```python
from build123d import *

# Parameters (mm, degrees)
SALIENTE_EXTRUIR1_DEPTH = 20
CORTAR_EXTRUIR1_DEPTH   = 20
CROQUIS3_W              = 4
CROQUIS3_H              = 20
SALIENTE_EXTRUIR2_DEPTH = 5


with BuildPart() as part:
    # Croquis1 → Saliente-Extruir1 (new body)
    with BuildSketch(Plane(origin=(0, 0, 0), x_dir=(1, 0, 0), z_dir=(0, 1, 0))):
        Polygon((-5, 19), (-2, 19), (-2, 3), (2, 3), (2, 19), (26, 19), (26, 16), (5, 16), (5, 0), (-5, 0), align=None)
    extrude(amount=SALIENTE_EXTRUIR1_DEPTH)

    # Croquis2 → Cortar-Extruir1 (cut)
    with BuildSketch(Plane.XY.offset(-16)):
        with BuildLine():
            Line((21.5, 16.5), (9.5, 16.5))
            ThreePointArc((9.5, 16.5), (8, 15), (9.5, 13.5))
            Line((9.5, 13.5), (21.5, 13.5))
            ThreePointArc((21.5, 13.5), (23, 15), (21.5, 16.5))
        make_face()
        with BuildLine():
            Line((21.5, 3.5), (9.5, 3.5))
            ThreePointArc((9.5, 3.5), (8, 5), (9.5, 6.5))
            Line((9.5, 6.5), (21.5, 6.5))
            ThreePointArc((21.5, 6.5), (23, 5), (21.5, 3.5))
        make_face()
    extrude(amount=-CORTAR_EXTRUIR1_DEPTH, mode=Mode.SUBTRACT)

    # Croquis3 → Saliente-Extruir2 (add)
    with BuildSketch(Plane(origin=(-2, 0, 0), x_dir=(0, 0, -1), z_dir=(1, 0, 0))):
        with Locations((17, 10)):
            Rectangle(CROQUIS3_W, CROQUIS3_H)
    extrude(amount=SALIENTE_EXTRUIR2_DEPTH)


solid = part.part
```
CAD build for the part. Positions are in the model's coordinates, mm. A direction names the side the tool comes from. Coordinates: 2 decimals unless noted, no trailing zeros. Order: outer loops, then holes, each group sorted by start corner. A loop starts at its lowest first (then second) coordinate and runs counter-clockwise, first axis right, second up. Notation, with made-up numbers: (32, 19) -> (51, 19) arc R24 ccw to (51, 58) -> close; hole circle Ø8 at (-39.75, -16). An arc over 180 degrees is marked (long way). Use one line per item in the form item = value. Start each with the question number.
1) Drop flat-ended pins along their axis: pin 1 (10 mm diameter, centred on x = 14.5, y = 8, fed in from +Z); pin 2 (5 mm diameter, centred on y = 7, z = -11.5, fed in from +X). Give the stop position or say it passes through.
2) Tool access for faces 1 (the flat face through (0, 10, -15)), 2 (the flat face through (16, 10, -16)), 3 (the flat face through (15, 6.5, -17)): list every direction of +Z, -Z, +X, -X, +Y, -Y with a clear straight run to the whole face (end or side of a thin tool).
3) Pull direction X, two halves, no side cores. Call faces 4 (the flat face through (-5, 10, -9)), 5 (the flat face through (15, 13.5, -17)), 6 (the flat face through (26, 10, -18)): +X half, -X half, draft (parallel to the pull), parting line (faces both ways), or undercut.
4) Drill centre lines: L1, parallel to X at y = 5, z = -8.5; L2, parallel to Z at x = -0.5, y = 1; L3, parallel to X at y = 13.5, z = -2. Where is each one in solid material? Low to high. Write a range as [from, to].
5) Band-saw the part on C-C on x = 15. Give the cut face in (y, z).
6) Band-saw the part on B-B on z = -6.5. Give the cut face in (x, y).
7) Band-saw the part on D-D on y = 11.5. Give the cut face in (x, z), then the cut area to 3 significant figures.
8) Band-saw the part on A-A on y = 15. Give the cut face in (x, z).
Entries:
q1.pin_1 = -16
q1.pin_2 = 5
q2.face_1 = +Y, -Y
q2.face_2 = +Z, +X, +Y, -Y
q2.face_3 = +Z, -Z
q3.face_4 = -X half
q3.face_5 = undercut
q3.face_6 = +X half
q4.L1 = [-5, -2], [2, 5]
q4.L2 = [-19, -15], [-3, 0]
q4.L3 = [-5, 5]
q5.outline = (0, -19) -> (3.5, -19) -> (3.5, -16) -> (0, -16) -> close; (6.5, -19) -> (13.5, -19) -> (13.5, -16) -> (6.5, -16) -> close; (16.5, -19) -> (20, -19) -> (20, -16) -> (16.5, -16) -> close
q6.outline = (-5, 0) -> (-2, 0) -> (-2, 20) -> (-5, 20) -> close; (2, 0) -> (5, 0) -> (5, 20) -> (2, 20) -> close
q7.outline = (-5, -19) -> (26, -19) -> (26, -16) -> (5, -16) -> (5, 0) -> (-5, 0) -> close; hole (-2, -15) -> (2, -15) -> (2, -3) -> (-2, -3) -> close
q7.area = 205 mm2
q8.outline = (-5, -19) -> (8, -19) -> (8, -16) -> (5, -16) -> (5, 0) -> (-5, 0) -> close; (23, -19) -> (26, -19) -> (26, -16) -> (23, -16) -> close; hole (-2, -15) -> (2, -15) -> (2, -3) -> (-2, -3) -> close
